CAD build for the part. Positions are in the model's coordinates, mm. A direction names the side the tool comes from. Round coordinates to 2 decimals unless told otherwise and drop trailing zeros. Loops run counter-clockwise (first coordinate to the right, second up) from the corner with the lowest first, then second, coordinate; pieces in that order, holes last.
from build123d import *

# Parameters (mm, degrees)
F0_W           = 50
F0_H           = 40
F1_DEPTH       = 50
F3_D           = 9
F3_CBORE_D     = 14.25
F3_CBORE_DEPTH = 8
F4_R           = 5


with BuildPart() as f1:
    # F0 (on Front) → F1 (new body)
    with BuildSketch(Plane.XZ):
        with Locations((25, 20)):
            Rectangle(F0_W, F0_H)
    extrude(amount=F1_DEPTH)

    # F3 (through all)
    with Locations(Plane.XZ.offset(50)):
        with Locations((27.4210199714, 20.3279424459)):
            CounterBoreHole(F3_D / 2, F3_CBORE_D / 2, F3_CBORE_DEPTH)

    # F4
    f4_edges = [f1.edges().sort_by_distance(p)[0] for p in [
        (25, -50, 40),
        (50, -50, 20),
        (50, -25, 40),
    ]]
    fillet(f4_edges, radius=F4_R)


solid = f1.part
Item 1: Flat gauge pins, fed straight in: P1, Ø7, axis at x = 27.42, z = 20.33, coming from the -Y side; P2, Ø4, axis at x = 30, z = 33, coming from the +Y side. Where does each tip first touch, or does it go through?
Verdict:
P1: passes through
P2: stops at y = 0
Item 2: Cut at A-A (x = 29). List the corners of the cut face in (y, z), plus the area to 3 significant figures.
Verdict:
outline: (-50, 0) - (0, 0) - (0, 16.11) - (-42, 16.11) - (-42, 13.38) - (-50, 13.38) - close; (-50, 27.28) - (-42, 27.28) - (-42, 24.54) - (0, 24.54) - (0, 40) - (-45, 40) arc R5 ccw to (-50, 35) - close
area: 1,530 mm2
Item 3: 3-axis set-ups, long thin cutter, end or side, ignore diameter. For faces 1 (the cylindrical face through (20.3, -46.1, 20.6)), 2 (the flat face through (22, -22, 40)): which of +Z, -Z, +X, -X, +Y, -Y reach the whole face in a straight line?
Verdict:
face 1: -Y
face 2: +Z, +X, -X, +Y, -Y
Item 4: Mould opens along X. For faces 3 (the cylindrical face through (31.917, -20.706, 20.526)), 4 (the cylindrical face through (48, -23, 39)), 5 (the flat face through (22, -50, 14)) say: released by +X, released by -X, zero draft, split by the parting line, or undercut.
Verdict:
face 3: undercut
face 4: released by +X
face 5: zero draft
Item 5: Cut at C-C (z = 15). List the corners of the cut face in (x, y).
Verdict:
outline: (0, -50) - (22.69, -50) - (22.69, -42) - (32.15, -42) - (32.15, -50) - (45, -50) arc R5 ccw to (50, -45) - (50, 0) - (0, 0) - close
Item 6: Cut at B-B (z = 19). List the corners of the cut face in (x, y).
Verdict:
outline: (0, -50) - (20.42, -50) - (20.42, -42) - (23.12, -42) - (23.12, 0) - (0, 0) - close; (31.72, -42) - (34.42, -42) - (34.42, -50) - (45, -50) arc R5 ccw to (50, -45) - (50, 0) - (31.72, 0) - close
Item 7: Cut at D-D (y = -6.5). List the corners of the cut face in (x, z).
Verdict:
outline: (0, 0) - (50, 0) - (50, 35) arc R5 ccw to (45, 40) - (0, 40) - close; hole circle Ø9 at (27.42, 20.33)
Item 8: Wall check: L1, parallel to Z at x = 27.5, y = -35.5; L2, parallel to Y at x = 33.5, z = 20.5; L3, parallel to X at y = -47.5, z = 21.5. Give the ranges that are in metal, low to high.
Verdict:
L1: z = 0 to 15.83, 24.83 to 40
L2: y = -42 to 0
L3: x = 0 to 20.39, 34.45 to 49.33
